```python
from build123d import *

# Parameters (mm, degrees)
SKETCH1_R                = 47.5
BOSS_EXTRUDE1_DEPTH      = 100
BOSS_EXTRUDE2_REACH      = 757.654
BOSS_EXTRUDE2_END_RADIUS = 47.5
SKETCH2_R                = 47.5
SKETCH2_R_2              = 40
BOSS_EXTRUDE4_REACH      = 661.36
SKETCH3_R                = 40
SKETCH4_R                = 25
CUT_EXTRUDE1_DEPTH       = 100


with BuildPart() as part:
    # Sketch1 → Boss-Extrude1 (new body)
    with BuildSketch(Plane.XY):
        Circle(SKETCH1_R)
    extrude(amount=BOSS_EXTRUDE1_DEPTH)

    # Boss-Extrude2: up to this cylinder (the profile starts outside it)
    boss_extrude2_end = Plane(origin=(0, 0, 96.156497), z_dir=(0, 0, -1)) * Cylinder(BOSS_EXTRUDE2_END_RADIUS, 1611.308, mode=Mode.PRIVATE)
    # Sketch2 → Boss-Extrude2 (add, up to the surface)
    with BuildSketch(Plane(origin=(700, 0, 0), x_dir=(0, 0, -1), z_dir=(1, 0, 0)), mode=Mode.PRIVATE) as boss_extrude2_sk1:
        with Locations((-50, 0)):
            Circle(SKETCH2_R)
        with Locations((-50, 0)):
            Circle(SKETCH2_R_2, mode=Mode.SUBTRACT)
    boss_extrude2_tool1 = extrude(boss_extrude2_sk1.sketch, amount=-BOSS_EXTRUDE2_REACH, mode=Mode.PRIVATE) - boss_extrude2_end
    add(boss_extrude2_tool1.solids().sort_by_distance((700, 0, 96.156497))[0])

    # Sketch3 → Boss-Extrude4 (add, up to next)
    with BuildSketch(Plane(origin=(50, 0, 0), x_dir=(0, 0, -1), z_dir=(1, 0, 0)), mode=Mode.PRIVATE) as boss_extrude4_sk1:
        with Locations((-50, 0)):
            Circle(SKETCH3_R)
    boss_extrude4_tool1 = extrude(boss_extrude4_sk1.sketch, amount=-BOSS_EXTRUDE4_REACH, mode=Mode.PRIVATE) - part.part
    add(boss_extrude4_tool1.solids().sort_by_distance((50, 0, 50))[0])

    # Sketch4 → Cut-Extrude1 (cut)
    with BuildSketch(Plane(origin=(0, 0, 0), x_dir=(-1, 0, 0), z_dir=(0, 0, -1))):
        Circle(SKETCH4_R)
    extrude(amount=-CUT_EXTRUDE1_DEPTH, mode=Mode.SUBTRACT)


solid = part.part
```
Source: CAD feature listing. Evaluate the final solid. Frame: model axes, mm. A direction names the side the tool comes from. Coordinates: 2 decimals unless noted, no trailing zeros. Loops run counter-clockwise (first coordinate to the right, second up) from the corner with the lowest first, then second, coordinate; pieces in that order, holes last. Notation, with made-up numbers: M 75,64 L 94,64 A32 cw 94,102 Z; hole C 82,-34.75 d7. An arc over 180 degrees is marked long. Put each result on its own line as item: value. Start each with the question number.
1) Cut plane C-C on x = 342.5. Return the cut outline in (y, z), then the cut area to 3 significant figures.
2) Ray query, L1, parallel to X at y = 1, z = 34; L2, parallel to Y at x = 613.5, z = 48; L3, parallel to Y at x = 18.5, z = 75. Return the intervals inside material, ascending. Write a range as from..to.
3) Cut plane B-B on z = 50. Return the cut outline in (x, y), then the cut area to 3 significant figures.
4) Contact query for flat-ended pins moving along their axis: pin 1 Ø6 at (x, z) = (321.5, 27.5) entering from -Y; pin 2 Ø6 at (y, z) = (2.5, 40) entering from +X; pin 3 Ø4 at (y, z) = (-37, 28) entering from -X. Output: stop coordinate, or through.
5) Cut plane A-A on y = 0. Return the cut outline in (x, z), then the cut area to 3 significant figures.
6) Cut plane D-D on y = -32.5. Return the cut outline in (x, z), then the cut area to 3 significant figures.
7) Reachability of faces 1 (the face through (50, 1, 51)), 2 (the face through (20, -20, 0)) from +Z, -Z, +X, -X, +Y, -Y: full face, straight path, thin tool, end or side. Return the list, or none.
8) Pull-direction query (Z, two-part tool) for faces 3 (the face through (379.55, 12.015, 11.847)), 4 (the face through (20, -20, 100)), 5 (the face through (354.9, 2.088, 97.454)); classes: pulls with the +Z half, pulls with the -Z half, needs draft (parallel to the pull), parting line crosses it, or undercut.
The answers:
1. outline: C 0,50 d95; hole C 0,50 d80
1. area: 2,060 mm²
2. L1: x = -47.49..-24.98, 24.98..50
2. L2: y = -47.46..-39.95, 39.95..47.46
2. L3: y = -43.75..-16.82, 16.82..43.75
3. outline: M 0,-47.5 L 700,-47.5 L 700,-40 L 50,-40 L 50,40 L 700,40 L 700,47.5 L 0,47.5 A47.5 ccw Z; hole C 0,0 d50
3. area: 16,100 mm²
4. pin 1: stops at y = -43.31
4. pin 2: stops at x = 50
4. pin 3: stops at x = -32.11
5. outline: M -47.5,0 L -25,0 L -25,100 L -47.5,100 Z; M 25,0 L 47.5,0 L 47.5,2.5 L 700,2.5 L 700,10 L 50,10 L 50,90 L 700,90 L 700,97.5 L 47.5,97.5 L 47.5,100 L 25,100 Z
5. area: 14,500 mm²
6. outline: M -34.64,0 L 34.64,0 L 34.64,15.36 L 700,15.36 L 700,26.68 L 50,26.68 L 50,73.32 L 700,73.32 L 700,84.64 L 34.64,84.64 L 34.64,100 L -34.64,100 Z
6. area: 22,700 mm²
7. face 1: +X
7. face 2: -Z, +X, -X, +Y, -Y
8. face 3: undercut
8. face 4: pulls with the +Z half
8. face 5: parting line crosses it
